```python
from build123d import *

# Parameters (mm, degrees)
F0_W     = 9
F0_H     = 85.5
F0_R     = 1.85
F1_DEPTH = 4.5
F2_R     = 2.3
F3_DEPTH = 5
F4_R     = 2.3
F5_DEPTH = 2.6
F6_R     = 3
F6_R_2   = 1.85
F7_DEPTH = 2


with BuildPart() as f1:
    # F0 (on Top) → F1 (new body)
    with BuildSketch(Plane.XY):
        Rectangle(F0_W, F0_H)
        with Locations((0, 7.25)):
            Circle(F0_R, mode=Mode.SUBTRACT)
        with Locations((0, 38.25)):
            Circle(F0_R, mode=Mode.SUBTRACT)
    extrude(amount=F1_DEPTH)

    # F2 (on face) → F3 (join)
    with BuildSketch(Plane.XZ.offset(42.75)):
        Polygon((5.144893, 5.634928), (6.799043, 8.605333), (3.3083, 14.44081), (-3.490743, 14.335477), (-6.799043, 8.394667), (-5.053671, 5.476928), (-4.5, 4.5), (4.5, 4.5), align=None)
        with Locations((0, 8.5)):
            Circle(F2_R, mode=Mode.SUBTRACT)
    extrude(amount=-F3_DEPTH)

    # F4 (on face) → F5 (cut)
    with BuildSketch(Plane.XZ.offset(42.75)):
        Polygon((4.387461, 8.559325), (2.142354, 12.329315), (-2.245107, 12.26999), (-4.387461, 8.440675), (-2.142354, 4.670685), (2.245107, 4.73001), align=None)
        with Locations((0, 8.5)):
            Circle(F4_R, mode=Mode.SUBTRACT)
    extrude(amount=-F5_DEPTH, mode=Mode.SUBTRACT)

    # F6 (on face) → F7 (cut)
    with BuildSketch(Plane.XY.offset(4.5)):
        with Locations((0, 38.25)):
            Circle(F6_R)
        with Locations((0, 38.25)):
            Circle(F6_R_2, mode=Mode.SUBTRACT)
        with Locations((0, 7.25)):
            Circle(F6_R)
        with Locations((0, 7.25)):
            Circle(F6_R_2, mode=Mode.SUBTRACT)
    extrude(amount=-F7_DEPTH, mode=Mode.SUBTRACT)


solid = f1.part
```
The listing builds one solid part. Answer for the finished solid, in the listing's coordinates (mm). A direction names the side the tool comes from. Coordinates: 2 decimals unless noted, no trailing zeros. Loops run counter-clockwise (first coordinate to the right, second up) from the corner with the lowest first, then second, coordinate; pieces in that order, holes last. Notation, with made-up numbers: M -22,78 L 33,78 A24 ccw 33,92 Z; hole C -23.5,87.25 d8. An arc over 180 degrees is marked long. Answer as a JSON object with one key per item and string values. Group by question number.
Item 1: Determine the mould class of faces 4 (the face through (-0.391, 41.224, 3.514)), 5 (the face through (-5.12, -40.28, 11.41)), 6 (the face through (0, 42.75, 2)) for opening direction Y: +Y half, -Y half, draft (parallel to the pull), parting line (faces both ways), or undercut.
Item 2: Section B-B (z = 7.25) is taken. Write down the section's boundary in (x, y).
Item 3: Each of these flat-tipped pins is pushed along its axis until it touches: P1, Ø3.5, axis at x = 0, y = 38.25, coming from the -Z side; P2, Ø3, axis at x = -1.5, y = 6, coming from the +Z side; P3, Ø6, axis at y = 13.5, z = 1.5, coming from the +X side; P4, Ø1.8, axis at x = -1.5, y = 37, coming from the +Z side. Where does it stop, or does it pass through?
Item 4: Consider L1, parallel to Y at x = 0, z = 3.95; L2, parallel to Y at x = 1, z = 3.25; L3, parallel to Y at x = -1.5, z = 13.75. Determine where each line is inside the solid, lowest interval first.
Item 5: Section C-C (y = 24.5) is taken. Write down the section's boundary in (x, z), and give its area (3 significant figures).
Item 6: Section A-A (y = 38.25) is taken. Write down the section's boundary in (x, z), and give its area (4 significant figures).
Item 7: Which of the six approach directions +Z, -Z, +X, -X, +Y, -Y give full straight-line access (tool end or side, diameter ignored) to faces 1 (the face through (-2, -37.75, 11)), 2 (the face through (2, -40.15, 10)), 3 (the face through (-2.997, 7.382, 3.514))?
Solved:
{
 "1": {"face 4": "undercut", "face 5": "draft", "face 6": "+Y half"},
 "2": {"outline": "M -6.11,-42.75 L -3.68,-42.75 L -3.68,-40.15 L -1.93,-40.15 L -1.93,-37.75 L -6.11,-37.75 Z; M 1.93,-40.15 L 3.65,-40.15 L 3.65,-42.75 L 6.04,-42.75 L 6.04,-37.75 L 1.93,-37.75 Z"},
 "3": {"P1": "passes through", "P2": "stops at z = 4.5", "P3": "stops at x = 4.5", "P4": "stops at z = 2.5"},
 "4": {"L1": "y = -42.75 to 4.25, 10.25 to 35.25, 41.25 to 42.75", "L2": "y = -42.75 to 4.42, 10.08 to 35.42, 41.08 to 42.75", "L3": "y = -42.75 to -37.75"},
 "5": {"outline": "M -4.5,0 L 4.5,0 L 4.5,4.5 L -4.5,4.5 Z", "area": "40.5 mm2"},
 "6": {"outline": "M -4.5,0 L -1.85,0 L -1.85,2.5 L -3,2.5 L -3,4.5 L -4.5,4.5 Z; M 1.85,0 L 4.5,0 L 4.5,4.5 L 3,4.5 L 3,2.5 L 1.85,2.5 Z", "area": "19.25 mm2"},
 "7": {"face 1": "+Z, +X, -X, +Y", "face 2": "-Y", "face 3": "+Z"}
}
